CAD build for the part. Positions are in the model's coordinates, mm. A direction names the side the tool comes from. Round coordinates to 2 decimals unless told otherwise and drop trailing zeros. Loops run counter-clockwise (first coordinate to the right, second up) from the corner with the lowest first, then second, coordinate; pieces in that order, holes last.
Autodesk Inventor part; units mm, degrees
ref_plane "YZ Plane" through (0, 0, 0) normal (1, 0, 0) x (0, 1, 0)
ref_plane "XZ Plane" through (0, 0, 0) normal (0, 1, 0) x (-1, 0, 0)
ref_plane "XY Plane" through (0, 0, 0) normal (0, 0, 1) x (1, 0, 0)
sketch "Sketch1" plane through (0, 0, 0) normal (0, 1, 0) x (-1, 0, 0)
  line L0 (-45, -29.5) -> (45, -29.5)
  line L1 (45, -29.5) -> (45, 29.5)
  line L2 (45, 29.5) -> (-45, 29.5)
  line L3 (-45, 29.5) -> (-45, -29.5)
  line L4 (-45, -29.5) -> (45, 29.5) construction
  line L5 (45, -29.5) -> (-45, 29.5) construction
  point P0 (0, 0)
  dimension "d0" = 59
  dimension "d1" = 90
extrude "Extrusion1" add sketch "Sketch1" along normal blind 17
sketch "Sketch2" plane through (0, 17, 0) normal (0, 1, 0) x (1, 0, 0)
  line L0 (-45, 29.5) -> (-45, -29.5)
  line L1 (-45, -29.5) -> (-29, -29.5)
  line L2 (-29, -29.5) -> (-29, 4.5)
  line L3 (-29, 4.5) -> (-45, 4.5)
  line L4 (-45, 4.5) -> (-45, -29.5)
  line L5 (45, -29.5) -> (-18, -29.5)
  line L6 (-18, -29.5) -> (-18, 4.5)
  line L7 (-18, 4.5) -> (45, 4.5)
  line L8 (45, 4.5) -> (45, -29.5)
  line L9 (45, 29.5) -> (-45, 29.5)
  line L10 (45, -29.5) -> (45, 29.5)
  line L11 (-45, -29.5) -> (45, -29.5)
  point P0 (0, 0)
  dimension "d4" = 25
  dimension "d5" = 25
  dimension "d6" = 16
  dimension "d7" = 63
extrude "Extrusion2" cut sketch "Sketch2" against normal blind 12 contours L3 L2 L1 L0 | L8 L5 L6 L7
sketch "Sketch3" plane through (0, 0, 0) normal (0, -1, 0) x (1, 0, 0)
  line L0 (-41, 4.1) -> (43, 4.1)
  line L1 (-45, -29.5) -> (-45, 29.5)
  line L2 (45, 29.5) -> (45, -29.5)
  line L3 (-45, 29.5) -> (45, 29.5)
  point P0 (0, 0)
  dimension "d10" = 4
  dimension "d11" = 2
  dimension "d12" = 25.4
hole "Hole1" at (-41, 0, 4.1) at (43, 0, 4.1) direction (0, 1, 0) diameter 3.2 end through all
equation "\"d5\" = d4"
properties part number "Eth_Switch"
Item 1: Cut at D-D (z = 20). List the corners of the cut face in (x, y).
Verdict:
outline: (-45, 0) - (45, 0) - (45, 5) - (-18, 5) - (-18, 17) - (-29, 17) - (-29, 5) - (-45, 5) - close
Item 2: Cut at C-C (y = 15.25). List the corners of the cut face in (x, z), plus the area to 3 significant figures.
Verdict:
outline: (-45, -29.5) - (45, -29.5) - (45, -4.5) - (-18, -4.5) - (-18, 29.5) - (-29, 29.5) - (-29, -4.5) - (-45, -4.5) - close
area: 2,620 mm2
Item 3: Cut at A-A (z = 4.1). List the corners of the cut face in (x, y), plus the area to 3 significant figures.
Verdict:
outline: (-45, 0) - (-42.6, 0) - (-42.6, 5) - (-45, 5) - close; (-39.4, 0) - (41.4, 0) - (41.4, 5) - (-18, 5) - (-18, 17) - (-29, 17) - (-29, 5) - (-39.4, 5) - close; (44.6, 0) - (45, 0) - (45, 5) - (44.6, 5) - close
area: 550 mm2
Item 4: Cut at B-B (x = -41). List the corners of the cut face in (y, z), plus the area to 3 significant figures.
Verdict:
outline: (0, -29.5) - (17, -29.5) - (17, -4.5) - (5, -4.5) - (5, 2.5) - (0, 2.5) - close; (0, 5.7) - (5, 5.7) - (5, 29.5) - (0, 29.5) - close
area: 579 mm2
Item 5: Flat gauge pins, fed straight in: P1, Ø2, axis at y = 8, z = 1, coming from the -X side; P2, Ø3.5, axis at x = -41, z = 4.1, coming from the +Y side; P3, Ø3.5, axis at y = 9.5, z = 16, coming from the +X side. Where does each tip first touch, or does it go through?
Verdict:
P1: stops at x = -29
P2: stops at y = 5
P3: stops at x = -18
Item 6: 3-axis set-ups, long thin cutter, end or side, ignore diameter. For faces 1 (the flat face through (-37, 5, 12)), 2 (the flat face through (-0.6, 4.6, 29.5)), 3 (the flat face through (13, 11, -4.5)): which of +Z, -Z, +X, -X, +Y, -Y reach the whole face in a straight line?
Verdict:
face 1: +Z, -X, +Y
face 2: +Z, +X, -X, +Y, -Y
face 3: +Z, +X, +Y
Item 7: Mould opens along Z. For faces 4 (the flat face through (1, 8, -29.5)), 5 (the cylindrical face through (-39.58, 2.54, 3.36)), 6 (the flat face through (-29, 11, 13)) say: released by +Z, released by -Z, zero draft, split by the parting line, or undercut.
Verdict:
face 4: released by -Z
face 5: undercut
face 6: zero draft
Item 8: Wall check: L1, parallel to X at y = 3.7, z = 4.1; L2, parallel to Z at x = -41, y = 2.2; L3, parallel to Y at x = 18.5, z = 1. Give the ranges that are in metal, low to high.
Verdict:
L1: x = -45 to -42.6, -39.4 to 41.4, 44.6 to 45
L2: z = -29.5 to 2.5, 5.7 to 29.5
L3: y = 0 to 5
